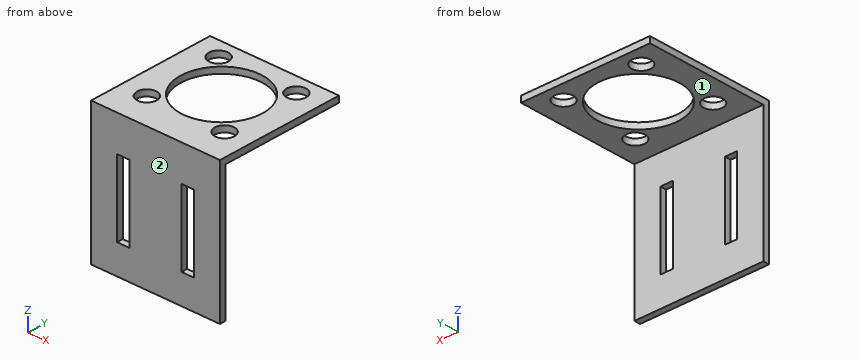
```python
from build123d import *

# Parameters (mm, degrees)
BOSS_EXTRUDE1_DEPTH     = 63
SKETCH2_R               = 4.75
SKETCH2_R_2             = 20
CUT_EXTRUDE1_DEPTH      = 35.80267333
CUT_EXTRUDE1_DEPTH_BACK = 34.19732667
SKETCH3_W               = 6
SKETCH3_H               = 36.550616257
CUT_EXTRUDE2_DEPTH      = 4


with BuildPart() as part:
    # Sketch1 → Boss-Extrude1 (new body)
    with BuildSketch(Plane(origin=(0, 0, 0), x_dir=(0, 0, -1), z_dir=(1, 0, 0))):
        Polygon((-31.80267333, 29.42384106), (-31.80267333, -30.57615894), (33.19732667, -30.57615894), (33.19732667, -33.57615894), (-34.80267333, -33.57615894), (-34.80267333, 29.42384106), align=None)
    extrude(amount=BOSS_EXTRUDE1_DEPTH)

    # Sketch2 → Cut-Extrude1 (cut, two sides)
    with BuildSketch(Plane.XY) as cut_extrude1_sk:
        with Locations((50.5, -17.57615894)):
            Circle(SKETCH2_R)
        with Locations((50.5, 20.42384106)):
            Circle(SKETCH2_R)
        with Locations((12.5, -17.57615894)):
            Circle(SKETCH2_R)
        with Locations((12.5, 20.42384106)):
            Circle(SKETCH2_R)
        with Locations((31.5, 1.42384106)):
            Circle(SKETCH2_R_2)
    extrude(amount=CUT_EXTRUDE1_DEPTH, mode=Mode.SUBTRACT)
    extrude(cut_extrude1_sk.sketch, amount=-CUT_EXTRUDE1_DEPTH_BACK, mode=Mode.SUBTRACT)

    # Sketch3 → Cut-Extrude2 (cut, through all)
    with BuildSketch(Plane(origin=(0, -30.57615894, 0), x_dir=(1, 0, 0), z_dir=(0, 1, 0))):
        with Locations((15.75, 0.697326671)):
            Rectangle(SKETCH3_W, SKETCH3_H)
        with Locations((47.25, 0.697326671)):
            Rectangle(SKETCH3_W, SKETCH3_H)
    extrude(amount=-CUT_EXTRUDE2_DEPTH, mode=Mode.SUBTRACT)


solid = part.part
```
Geometry: final body of the model. Coordinates: model frame, mm. Face numbers are marked on the shaded views. A direction names the side the tool comes from. Round coordinates to 2 decimals unless told otherwise and drop trailing zeros. Order: outer loops, then holes, each group sorted by start corner. A loop starts at its lowest first (then second) coordinate and runs counter-clockwise, first axis right, second up. Notation, with made-up numbers: (-8.75, 79.25) -> (23.25, 79.25) arc R17 cw to (23.25, 111.25) -> close; hole circle Ø5 at (-0.75, -36.5). An arc over 180 degrees is marked (long way). Use one line per item in the form item = value. Start each with the question number.
1. Cut plane D-D (x = 57). Return the cut outline in (y, z), then the cut area to 3 significant figures.
2. Cut plane A-A (z = -13). Return the cut outline in (x, y).
3. Cut plane C-C (y = -16.5). Return the cut outline in (x, z).
4. Line query: probe 1 along Y at (x, z) = (57, 0); probe 2 along Z at (x, y) = (8.5, -20.5). Output: solid intervals per line, ascending.
5. Cut plane B-B (x = 31.5). Return the cut outline in (y, z).
6. Reachability of the marked faces 1 and 2 from +Z, -Z, +X, -X, +Y, -Y: full face, straight path, thin tool, end or side. Return the list, or none.
7. Pin query (flat end, axial travel): pin 1 Ø7.5 at (x, y) = (12.5, 20.42) entering from +Z; pin 2 Ø2 at (x, z) = (49.5, -5.5) entering from +Y. Return the tip coordinate at first contact, or that it passes through.
Solution:
q1.outline = (-33.58, -33.2) -> (-30.58, -33.2) -> (-30.58, 31.8) -> (29.42, 31.8) -> (29.42, 34.8) -> (-33.58, 34.8) -> close
q1.area = 384 mm^2
q2.outline = (0, -33.58) -> (12.75, -33.58) -> (12.75, -30.58) -> (0, -30.58) -> close; (18.75, -33.58) -> (44.25, -33.58) -> (44.25, -30.58) -> (18.75, -30.58) -> close; (50.25, -33.58) -> (63, -33.58) -> (63, -30.58) -> (50.25, -30.58) -> close
q3.outline = (0, 31.8) -> (7.87, 31.8) -> (7.87, 34.8) -> (0, 34.8) -> close; (17.13, 31.8) -> (22.63, 31.8) -> (22.63, 34.8) -> (17.13, 34.8) -> close; (40.37, 31.8) -> (45.87, 31.8) -> (45.87, 34.8) -> (40.37, 34.8) -> close; (55.13, 31.8) -> (63, 31.8) -> (63, 34.8) -> (55.13, 34.8) -> close
q4.probe_1 = -33.58 to -30.58
q4.probe_2 = 31.8 to 34.8
q5.outline = (-33.58, -33.2) -> (-30.58, -33.2) -> (-30.58, 31.8) -> (-18.58, 31.8) -> (-18.58, 34.8) -> (-33.58, 34.8) -> close; (21.42, 31.8) -> (29.42, 31.8) -> (29.42, 34.8) -> (21.42, 34.8) -> close
q6.face_1 = -Z, +X, -X, +Y
q6.face_2 = +Z, -Z, +X, -X, -Y
q7.pin_1 = through
q7.pin_2 = -30.58
